Verification items for the finished model (mm, model axes). Face numbers are marked on the shaded views. Coordinates: 2 decimals unless noted, no trailing zeros. Order: outer loops, then holes, each group sorted by start corner. A loop starts at its lowest first (then second) coordinate and runs counter-clockwise, first axis right, second up. Notation, with made-up numbers: M 82,-37 L 112,-37 A23 ccw 112,-1 Z; hole C 67.5,-39.5 d7. An arc over 180 degrees is marked long. Return JSON: item names as keys, results as strings.
```python
from build123d import *

# Parameters (mm, degrees)
SKETCH2_W                       = 50
SKETCH2_H                       = 20
BOSS_EXTRUDE1_DEPTH             = 6.35
M5_CLEARANCE_HOLE1_D            = 5.5
TAP_DRILL_FOR_M3X0_5_TAP1_D     = 2.5
TAP_DRILL_FOR_M3X0_5_TAP1_DEPTH = 6.35
TAP_DRILL_FOR_M3X0_5_TAP1_TIP   = 0.751075774
FILLET1_R                       = 7.5


with BuildPart() as part:
    # Sketch2 → Boss-Extrude1 (new body)
    with BuildSketch(Plane(origin=(0, 0, 0), x_dir=(1, 0, 0), z_dir=(0, 1, 0))):
        with Locations((25, 10)):
            Rectangle(SKETCH2_W, SKETCH2_H)
    extrude(amount=BOSS_EXTRUDE1_DEPTH)

    # M5 Clearance Hole1 (through all)
    with Locations(Plane(origin=(8, 6.35, -10), x_dir=(0, 0, 1), z_dir=(0, 1, 0))):
        with Locations((0, 0), (0, 15)):
            Hole(M5_CLEARANCE_HOLE1_D / 2)

    # Tap Drill for M3x0.5 Tap1
    with Locations(Plane(origin=(45, 6.35, -10), x_dir=(0, 0, 1), z_dir=(0, 1, 0))):
        with Locations((0, 0)):
            Hole(TAP_DRILL_FOR_M3X0_5_TAP1_D / 2, depth=TAP_DRILL_FOR_M3X0_5_TAP1_DEPTH)
            with Locations((0, 0, -(TAP_DRILL_FOR_M3X0_5_TAP1_DEPTH + TAP_DRILL_FOR_M3X0_5_TAP1_TIP / 2))):  # 118° drill point
                Cone(0, TAP_DRILL_FOR_M3X0_5_TAP1_D / 2, TAP_DRILL_FOR_M3X0_5_TAP1_TIP, mode=Mode.SUBTRACT)

    # Fillet1
    fillet1_edges = [part.edges().sort_by_distance(p)[0] for p in [
        (0, 3.175, -20),
        (50, 3.175, -20),
        (50, 3.175, 0),
        (0, 3.175, 0),
    ]]
    fillet(fillet1_edges, radius=FILLET1_R)


solid = part.part
```
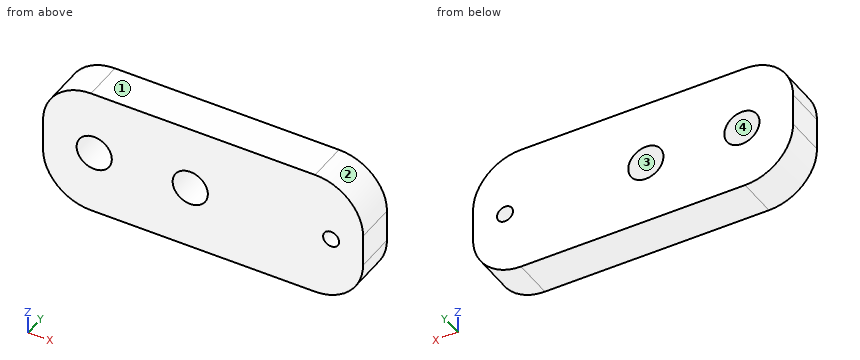
Q1. Draft check along X on the marked faces 1, 2, 3 and 4. Enter one of: pulls with the +X half, pulls with the -X half, needs draft (parallel to the pull), parting line crosses it, or undercut.
Values:
{"face 1": "needs draft", "face 2": "pulls with the +X half", "face 3": "undercut", "face 4": "undercut"}
Q2. Cross-section at B-B, the plane z = -10. Record the boundary of the cut face in (x, y), and give its area (3 significant figures).
Values:
{"outline": "M 0,0 L 5.25,0 L 5.25,6.35 L 0,6.35 Z; M 10.75,0 L 20.25,0 L 20.25,6.35 L 10.75,6.35 Z; M 25.75,0 L 43.75,0 L 43.75,6.35 L 25.75,6.35 Z; M 46.25,0 L 50,0 L 50,6.35 L 46.25,6.35 Z", "area": "232 mm^2"}
Q3. Cross-section at D-D, the plane x = 45. Record the boundary of the cut face in (y, z).
Values:
{"outline": "M 0,-19.57 L 6.35,-19.57 L 6.35,-11.25 L 0,-11.25 Z; M 0,-8.75 L 6.35,-8.75 L 6.35,-0.43 L 0,-0.43 Z"}
Q4. Material ranges on line 1 along X through (y, z) = (1.5, -10); line 2 along X through (y, z) = (5.25, -10.5); line 3 along Z through (x, y) = (46, 1.5), recorded low to high.
Values:
{"line 1": "0 to 5.25, 10.75 to 20.25, 25.75 to 43.75, 46.25 to 50", "line 2": "0 to 5.3, 10.7 to 20.3, 25.7 to 43.85, 46.15 to 50", "line 3": "-19.13 to -10.75, -9.25 to -0.87"}
Q5. Cross-section at C-C, the plane y = 3. Record the boundary of the cut face in (x, z).
Values:
{"outline": "M 0,-12.5 A7.5 ccw 7.5,-20 L 42.5,-20 A7.5 ccw 50,-12.5 L 50,-7.5 A7.5 ccw 42.5,0 L 7.5,0 A7.5 ccw 0,-7.5 Z; hole C 8,-10 d5.5; hole C 23,-10 d5.5; hole C 45,-10 d2.5"}
Q6. Go/stop test with a flat-tipped pin: pin 1 (10 mm diameter, centred on x = 22.5, z = -14.5, fed in from -Y). Record where the tip stops, or that it passes through.
Values:
{"pin 1": "y = 0"}
Q7. Cross-section at A-A, the plane x = 8. Record the boundary of the cut face in (y, z), and give its area (3 significant figures).
Values:
{"outline": "M 0,-20 L 6.35,-20 L 6.35,-12.75 L 0,-12.75 Z; M 0,-7.25 L 6.35,-7.25 L 6.35,0 L 0,0 Z", "area": "92.1 mm^2"}
